The listing builds one solid part. Answer for the finished solid, in the listing's coordinates (mm). A direction names the side the tool comes from. Coordinates: 2 decimals unless noted, no trailing zeros. Order: outer loops, then holes, each group sorted by start corner. A loop starts at its lowest first (then second) coordinate and runs counter-clockwise, first axis right, second up. Notation, with made-up numbers: (-26.75, 17.25) -> (-0.75, 17.25) arc R29 ccw to (-0.75, 44.25) -> close; hole circle Ø3 at (28, 54.5). An arc over 180 degrees is marked (long way). Answer in a Markdown table with one row per item.
```python
from build123d import *

# Parameters (mm, degrees)
ESQUISSE1_W             = 45.3
ESQUISSE1_H             = 14
BOSS_EXTRU_1_DEPTH      = 0.8
ESQUISSE2_W             = 44
ESQUISSE2_H             = 14
BOSS_EXTRU_2_DEPTH      = 5
ENL_V_MAT_EXTRU_1_DEPTH = 57


with BuildPart() as part:
    # Esquisse1 → Boss.-Extru.1 (new body)
    with BuildSketch(Plane.XY):
        Rectangle(ESQUISSE1_W, ESQUISSE1_H)
    extrude(amount=BOSS_EXTRU_1_DEPTH)

    # Esquisse2 → Boss.-Extru.2 (add)
    with BuildSketch(Plane.XY.offset(0.8)):
        Rectangle(ESQUISSE2_W, ESQUISSE2_H)
    extrude(amount=BOSS_EXTRU_2_DEPTH)

    # Esquisse4 → Enlèv. mat.-Extru.1 (cut)
    with BuildSketch(Plane.ZY.offset(22)):
        with BuildLine():
            Line((1.29, 7), (3.29, -3.15))
            Line((3.29, -3.15), (3.29, -4.5))
            ThreePointArc((3.29, -4.5), (2.561300162, -6.264234962), (0.8, -7))
            Line((0.8, -7), (9.633506855, -10.676835967))
            Line((9.633506855, -10.676835967), (7.497371295, 9.595509349))
            Line((7.497371295, 9.595509349), (1.29, 7))
        make_face()
    extrude(amount=-ENL_V_MAT_EXTRU_1_DEPTH, mode=Mode.SUBTRACT)


solid = part.part
```
(1) A cutting plane is placed at B-B, the plane y = 0. Determine the outline of the cut face in (x, z), then the cut area to 3 significant figures.
Check values:
| item | result |
|---|---|
| outline | (-22.65, 0) -> (22.65, 0) -> (22.65, 0.8) -> (22, 0.8) -> (22, 2.67) -> (-22, 2.67) -> (-22, 0.8) -> (-22.65, 0.8) -> close |
| area | 118 mm² |
(2) Flat-ended cylindrical pins translate along their axes: pin 1 (0.5 mm diameter, centred on x = 22.5, y = 3.5, fed in from +Z); pin 2 (8 mm diameter, centred on x = -16.5, y = 5, fed in from -Z); pin 3 (0.7 mm diameter, centred on y = 0, z = 2, fed in from -X); pin 4 (1 mm diameter, centred on y = -4, z = 1.5, fed in from +X). Find the tip coordinate at first contact, or state that the pin passes through.
Check values:
| item | result |
|---|---|
| pin 1 | z = 0.8 |
| pin 2 | z = 0 |
| pin 3 | x = -22 |
| pin 4 | x = 22 |
(3) Find the intervals of material crossed by line 1 along X through (y, z) = (-3.75, 1.6); line 2 along Z through (x, y) = (-17, 0.25); line 3 along Z through (x, y) = (19, 2.75), in increasing order. Write a range as from..to.
Check values:
| item | result |
|---|---|
| line 1 | -22..22 |
| line 2 | 0..2.62 |
| line 3 | 0..2.13 |
(4) A cutting plane is placed at C-C, the plane z = 1.7. Determine the outline of the cut face in (x, y).
Check values:
| item | result |
|---|---|
| outline | (-22, -6.83) -> (22, -6.83) -> (22, 4.92) -> (-22, 4.92) -> close |
(5) Which of the six approach directions +Z, -Z, +X, -X, +Y, -Y give full straight-line access (tool end or side, diameter ignored) to faces 1 (the flat face through (0, 7, 1)), 2 (the flat face through (-22, -2, 2)), 3 (the flat face through (22, -2, 2))?
Check values:
| item | result |
|---|---|
| face 1 | +Z, -Z, +X, -X, +Y |
| face 2 | +Z, -X, +Y, -Y |
| face 3 | +Z, +X, +Y, -Y |
(6) A cutting plane is placed at A-A, the plane x = -5. Determine the outline of the cut face in (y, z), then the cut area to 3 significant figures.
Check values:
| item | result |
|---|---|
| outline | (-7, 0) -> (7, 0) -> (7, 1.29) -> (-3.15, 3.29) -> (-4.5, 3.29) arc R2.5 ccw to (-7, 0.8) -> close |
| area | 34.6 mm² |
(7) A cutting plane is placed at D-D, the plane y = 2.75. Determine the outline of the cut face in (x, z).
Check values:
| item | result |
|---|---|
| outline | (-22.65, 0) -> (22.65, 0) -> (22.65, 0.8) -> (22, 0.8) -> (22, 2.13) -> (-22, 2.13) -> (-22, 0.8) -> (-22.65, 0.8) -> close |
